```python
from build123d import *

# Parameters (mm, degrees)
SKETCH309_R      = 1
EXTRUDE165_DEPTH = 2
SKETCH310_R      = 1
EXTRUDE164_DEPTH = 2
SKETCH307_R      = 1
EXTRUDE166_DEPTH = 2
SKETCH308_R      = 1
EXTRUDE163_DEPTH = 2
SKETCH314_R      = 0.635
EXTRUDE161_DEPTH = 2
SKETCH313_R      = 0.635
EXTRUDE159_DEPTH = 2
SKETCH315_R      = 0.635
EXTRUDE160_DEPTH = 2
SKETCH312_R      = 0.635
EXTRUDE162_DEPTH = 2
EXTRUDE_DEPTH    = 1.6


with BuildPart() as extrude165:
    # Sketch309 → Extrude165 (new body)
    with BuildSketch(Plane(origin=(1.17, 48.67, 0), x_dir=(1, 0, 0), z_dir=(0, 0, 1))):
        Circle(SKETCH309_R)
    extrude(amount=EXTRUDE165_DEPTH)


with BuildPart() as extrude164:
    # Sketch310 → Extrude164 (new body)
    with BuildSketch(Plane(origin=(52.17, 48.67, 0), x_dir=(1, 0, 0), z_dir=(0, 0, 1))):
        Circle(SKETCH310_R)
    extrude(amount=EXTRUDE164_DEPTH)


with BuildPart() as extrude166:
    # Sketch307 → Extrude166 (new body)
    with BuildSketch(Plane(origin=(1.17, 4.67, 0), x_dir=(1, 0, 0), z_dir=(0, 0, 1))):
        Circle(SKETCH307_R)
    extrude(amount=EXTRUDE166_DEPTH)


with BuildPart() as fusion042:
    # Sketch308 → Extrude163 (new body)
    with BuildSketch(Plane(origin=(52.17, 4.67, 0), x_dir=(1, 0, 0), z_dir=(0, 0, 1))):
        Circle(SKETCH308_R)
    extrude(amount=EXTRUDE163_DEPTH)

    # Fusion042: union Extrude165, Extrude164, Extrude166
    add(extrude165.part)
    add(extrude164.part)
    add(extrude166.part)


with BuildPart() as extrude161:
    # Sketch314 → Extrude161 (new body)
    with BuildSketch(Plane(origin=(23.6, -47.63, 13), x_dir=(1, 0, 0), z_dir=(0, 0, 1))):
        with Locations((10.16, 50.165)):
            Circle(SKETCH314_R)
        with Locations((7.62, 50.165)):
            Circle(SKETCH314_R)
        with Locations((12.7, 50.165)):
            Circle(SKETCH314_R)
        with Locations((15.24, 50.165)):
            Circle(SKETCH314_R)
        with Locations((17.78, 50.165)):
            Circle(SKETCH314_R)
        with Locations((20.32, 50.165)):
            Circle(SKETCH314_R)
        with Locations((22.86, 50.165)):
            Circle(SKETCH314_R)
        with Locations((25.4, 50.165)):
            Circle(SKETCH314_R)
    extrude(amount=EXTRUDE161_DEPTH)


with BuildPart() as extrude159:
    # Sketch313 → Extrude159 (new body)
    with BuildSketch(Plane(origin=(-3.3, -47.63, 13), x_dir=(1, 0, 0), z_dir=(0, 0, 1))):
        with Locations((10.16, 50.165)):
            Circle(SKETCH313_R)
        with Locations((7.62, 50.165)):
            Circle(SKETCH313_R)
        with Locations((12.7, 50.165)):
            Circle(SKETCH313_R)
        with Locations((15.24, 50.165)):
            Circle(SKETCH313_R)
        with Locations((17.78, 50.165)):
            Circle(SKETCH313_R)
        with Locations((20.32, 50.165)):
            Circle(SKETCH313_R)
        with Locations((22.86, 50.165)):
            Circle(SKETCH313_R)
        with Locations((25.4, 50.165)):
            Circle(SKETCH313_R)
        with Locations((27.94, 50.165)):
            Circle(SKETCH313_R)
        with Locations((30.48, 50.165)):
            Circle(SKETCH313_R)
    extrude(amount=EXTRUDE159_DEPTH)


with BuildPart() as extrude160:
    # Sketch315 → Extrude160 (new body)
    with BuildSketch(Plane(origin=(23.62, 0.63, 13), x_dir=(1, 0, 0), z_dir=(0, 0, 1))):
        with Locations((12.7, 50.165)):
            Circle(SKETCH315_R)
        with Locations((15.24, 50.165)):
            Circle(SKETCH315_R)
        with Locations((17.78, 50.165)):
            Circle(SKETCH315_R)
        with Locations((20.32, 50.165)):
            Circle(SKETCH315_R)
        with Locations((22.86, 50.165)):
            Circle(SKETCH315_R)
        with Locations((25.4, 50.165)):
            Circle(SKETCH315_R)
    extrude(amount=EXTRUDE160_DEPTH)


with BuildPart() as fusion:
    # Sketch312 → Extrude162 (new body)
    with BuildSketch(Plane(origin=(0.75, 0.63, 13), x_dir=(1, 0, 0), z_dir=(0, 0, 1))):
        with Locations((12.7, 50.165)):
            Circle(SKETCH312_R)
        with Locations((15.24, 50.165)):
            Circle(SKETCH312_R)
        with Locations((17.78, 50.165)):
            Circle(SKETCH312_R)
        with Locations((20.32, 50.165)):
            Circle(SKETCH312_R)
        with Locations((22.86, 50.165)):
            Circle(SKETCH312_R)
        with Locations((25.4, 50.165)):
            Circle(SKETCH312_R)
        with Locations((27.94, 50.165)):
            Circle(SKETCH312_R)
        with Locations((30.48, 50.165)):
            Circle(SKETCH312_R)
    extrude(amount=EXTRUDE162_DEPTH)

    # Fusion: union Extrude161, Extrude159, Extrude160
    add(extrude161.part)
    add(extrude159.part)
    add(extrude160.part)


with BuildPart() as fusion_1:
    # Fusion placement: moved
    add(fusion.part.moved(Location((0, 0, -13))))


with BuildPart() as obj1:
    # Sketch311 → Extrude (new body)
    with BuildSketch(Plane.XY):
        with BuildLine():
            Line((0, 53.34), (53.340001, 53.34))
            ThreePointArc((55.88, 50.8), (55.136052, 52.596051), (53.340001, 53.34))
            Line((55.88, 50.8), (55.88, 2.54))
            ThreePointArc((53.340001, 0), (55.136052, 0.743949), (55.88, 2.54))
            Line((0, 0), (53.340001, 0))
            ThreePointArc((-2.54, 2.540001), (-1.796052, 0.743949), (0, 0))
            Line((-2.54, 50.8), (-2.54, 2.540001))
            ThreePointArc((0, 53.34), (-1.796051, 52.596051), (-2.54, 50.8))
        make_face()
    extrude(amount=EXTRUDE_DEPTH)

    # Cut070: cut Fusion
    add(fusion_1.part, mode=Mode.SUBTRACT)

    # Cut071: cut Fusion042
    add(fusion042.part, mode=Mode.SUBTRACT)


solid = obj1.part
```
Geometry check sheet. Reference: the model listing, model coordinates, mm. Coordinates: 2 decimals unless noted, no trailing zeros. Loops run counter-clockwise (first coordinate to the right, second up) from the corner with the lowest first, then second, coordinate; pieces in that order, holes last.
Item 1: Release check for a two-part mould opening along X. For faces 1 (the face through (27, 27, 1.6)), 2 (the face through (-1.776, 52.616, 0.789)), 3 (the face through (21.596, 2.149, 0.789)) record: released by +X, released by -X, zero draft, split by the parting line, or undercut.
Item 2: Sectioned sample at B-B, the plane z = 0.7. Count the separate pieces of the cut face and the enclosed holes in it, then the cut area to 3 significant figures.
Item 3: Go/stop test with a flat-tipped pin: pin 1 Ø2 at (x, y) = (43.92, 2.535) entering from +Z. Record where the tip stops, or that it passes through.
Item 4: Thickness scan on line 1 (Y direction, x = 41.38, z = 1.2); line 2 (X direction, y = 4.67, z = 0.5); line 3 (Y direction, x = 52, z = 1.4). Record the ranges inside material, lowest first.
Item 5: Sectioned sample at A-A, the plane x = 11.94. Record the boundary of the cut face in (y, z).
Check result:
1. face 1: zero draft
1. face 2: released by -X
1. face 3: undercut
2. separate pieces: 1
2. enclosed holes: 36
2. area: 3,060 mm2
3. pin 1: stops at z = 1.6
4. line 1: y = 0 to 1.9, 3.17 to 50.16, 51.43 to 53.34
4. line 2: x = -2.54 to 0.17, 2.17 to 51.17, 53.17 to 55.88
4. line 3: y = 0 to 3.68, 5.66 to 47.68, 49.66 to 53.34
5. outline: (0, 0) - (1.9, 0) - (1.9, 1.6) - (0, 1.6) - close; (3.17, 0) - (53.34, 0) - (53.34, 1.6) - (3.17, 1.6) - close
